Job drawing, mm, ordinate dimensions from the low corner. One solid piece. A direction names the side the tool comes from. Coordinates: 2 decimals unless noted, no trailing zeros. Write each loop counter-clockwise with the first axis right and the second up, starting at its lowest first coordinate (ties: lowest second). Pieces come first, ordered by that corner, then holes. Notation, with made-up numbers: (42, 47.5) - (84, 47.5) arc R22 cw to (84, 65.5) - close; hole circle Ø1 at (3.5, 57.25). An arc over 180 degrees is marked (long way). Put each result on its own line as item: value. Start each with the question number.
1. Drill centre lines: L1, parallel to Z at x = 8.5, y = 8.5 (1 decimal); L2, parallel to Y at x = 48, z = 35 (1 decimal). Where is each one in solid material? Low to high. Write a range as from..to.
2. Saw through at A-A, the plane z = 38.1. Write the cut outline in (x, y) (1 decimal), plus the area to 3 significant figures.
3. Saw through at C-C, the plane x = 41. Write the cut outline in (y, z) (1 decimal).
4. Saw through at D-D, the plane y = 40.5. Write the cut outline in (x, z) (1 decimal), plus the area to 3 significant figures.
5. Which spindle directions (+Z, -Z, +X, -X, +Y, -Y) get a long thin tool onto all of the face, cutting with end or side? Do the marked faces 1 and 2. Say none if no direction does.
6. Drop flat-ended pins along their axis: P1, Ø6, axis at x = 43.5, z = 23.5, coming from the -Y side; P2, Ø8, axis at x = 29.76, y = 32.84, coming from the -Z side (1 decimal); P3, Ø4, axis at y = 21.5, z = 17.5, coming from the -X side (1 decimal). Give the stop position or say it passes through.
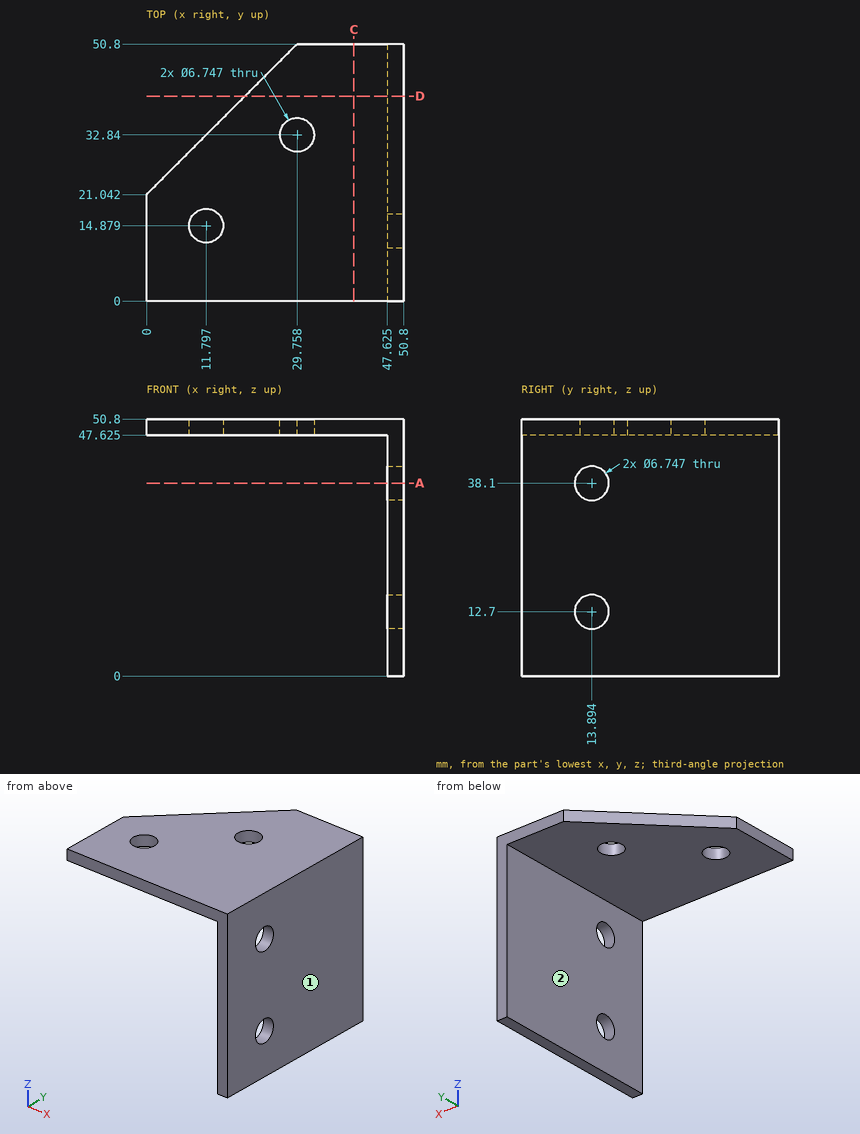
Final values:
1. L1: z = 47.6..50.8
1. L2: y = 0..12.6, 15.2..50.8
2. outline: (47.6, 0) - (50.8, 0) - (50.8, 10.5) - (47.6, 10.5) - close; (47.6, 17.3) - (50.8, 17.3) - (50.8, 50.8) - (47.6, 50.8) - close
2. area: 140 mm²
3. outline: (0, 47.6) - (50.8, 47.6) - (50.8, 50.8) - (0, 50.8) - close
4. outline: (19.5, 47.6) - (47.6, 47.6) - (47.6, 0) - (50.8, 0) - (50.8, 50.8) - (19.5, 50.8) - close
4. area: 251 mm²
5. face 1: +Z, -Z, +X, +Y, -Y
5. face 2: -Z, -X, +Y, -Y
6. P1: passes through
6. P2: stops at z = 47.6
6. P3: stops at x = 47.6
